from build123d import *

# Parameters (mm, degrees)
SKETCH1_W           = 71
SKETCH1_H           = 20
BOSS_EXTRUDE1_DEPTH = 6
CUT_EXTRUDE1_DEPTH  = 7


with BuildPart() as part:
    # Sketch1 → Boss-Extrude1 (new body)
    with BuildSketch(Plane(origin=(0, 0, 0), x_dir=(1, 0, 0), z_dir=(0, 1, 0))):
        Rectangle(SKETCH1_W, SKETCH1_H)
    extrude(amount=BOSS_EXTRUDE1_DEPTH)

    # Sketch4 → Cut-Extrude1 (cut, through all)
    with BuildSketch(Plane.XZ):
        Polygon((-35.5, 5), (-29.5, 5), (-29.5, 0), (-29.5, -5), (-35.5, -5), align=None)
    extrude(amount=-CUT_EXTRUDE1_DEPTH, mode=Mode.SUBTRACT)


solid = part.part
Part model, mm, in its own coordinate system. A direction names the side the tool comes from. Coordinates: 2 decimals unless noted, no trailing zeros. Loops run counter-clockwise (first coordinate to the right, second up) from the corner with the lowest first, then second, coordinate; pieces in that order, holes last. Notation, with made-up numbers: M 21,-5.5 L 52,-5.5 A21 ccw 52,0.5 Z; hole C -20,23 d10. An arc over 180 degrees is marked long. Use a Markdown table: item, result. Add a question column.
Q1. Cut at A-A (y = 2.5). Write the cut outline in (x, z), and give its area (3 significant figures).
Q2. Which spindle directions (+Z, -Z, +X, -X, +Y, -Y) get a long thin tool onto all of the face, cutting with end or side? Do faces 1 (the flat face through (-32, 3, -5)), 2 (the flat face through (0, 0, 0)). Say none if no direction does.
Q3. Pin check, flat tip, straight feed: P1, Ø3, axis at y = 4, z = -1.5, coming from the -X side. Stop position of the tip, or through.
Q4. Cut at B-B (z = 1.25). Write the cut outline in (x, y), and give its area (3 significant figures).
Q5. Mould opens along Z. For faces 3 (the flat face through (0, 3, -10)), 4 (the flat face through (-29.5, 3, 0)), 5 (the flat face through (0, 3, 10)), 6 (the flat face through (-35.5, 3, 8)) say: +Z half, -Z half, draft (parallel to the pull), parting line (faces both ways), or undercut.
Q6. Probe L1, parallel to Z at x = -30, y = 2.75; L2, parallel to X at y = 1.9, z = -3. List the from-to ranges inside material, lowest first.
Worked out:
| question | item | result |
|---|---|---|
| 1 | outline | M -35.5,-10 L 35.5,-10 L 35.5,10 L -35.5,10 L -35.5,5 L -29.5,5 L -29.5,-5 L -35.5,-5 Z |
| 1 | area | 1,360 mm2 |
| 2 | face 1 | -X, +Y, -Y |
| 2 | face 2 | +Z, -Z, +X, -X, -Y |
| 3 | P1 | stops at x = -29.5 |
| 4 | outline | M -29.5,0 L 35.5,0 L 35.5,6 L -29.5,6 Z |
| 4 | area | 390 mm2 |
| 5 | face 3 | -Z half |
| 5 | face 4 | undercut |
| 5 | face 5 | +Z half |
| 5 | face 6 | draft |
| 6 | L1 | z = -10 to -5, 5 to 10 |
| 6 | L2 | x = -29.5 to 35.5 |
